Source: CAD feature listing. Evaluate the final solid. Frame: model axes, mm. Face numbers are marked on the shaded views. Give positions to 0.01 mm unless a question says otherwise; leave off trailing zeros. Order: outer loops, then holes, each group sorted by start corner. A loop starts at its lowest first (then second) coordinate and runs counter-clockwise, first axis right, second up. Notation, with made-up numbers: (-30.75, 55.5) - (-3.75, 55.5) arc R23 ccw to (-3.75, 79.5) - close; hole circle Ø6 at (-27.75, 15). An arc over 180 degrees is marked (long way). Write each question's results on one line, items separated by ' | '. Start each with the question number.
Item 1: Mould query, pull axis X, two halves, no side actions, for the marked faces 1, 2 and 3. Classes: released by +X, released by -X, zero draft, split by the parting line, or undercut.
Item 2: Contact query for a flat-ended pin moving along its axis: pin 1 Ø5 at (x, z) = (-0.5, 1.5) entering from -Y. Output: stop coordinate, or through.
Item 3: Section A-A on z = 0. Output: boundary loops of the cut face in (x, y), and give its area (3 significant figures).
Item 4: Section B-B on y = 1.7. Output: boundary loops of the cut face in (x, z), and give its area (3 significant figures).
Item 5: Line query: line 1 along X through (y, z) = (3.45, 0); line 2 along Z through (x, y) = (-1, 2.85); line 3 along Z through (x, y) = (0.5, 1.2). Output: solid intervals per line, ascending.
```python
from build123d import *

# Parameters (mm, degrees)
BODY_SKETCH_R   = 5
BODY_SKETCH_R_2 = 2.25
BODY_DEPTH      = 5
CHAMFERS_SIZE   = 0.4


with BuildPart() as part:
    # body_sketch → body (new body)
    with BuildSketch(Plane(origin=(0, 0, 0), x_dir=(1, 0, 0), z_dir=(0, 1, 0))):
        with Locations(Location((0, 0, 0), (0, 0, 270))):
            Circle(BODY_SKETCH_R)
        with Locations(Location((0, 0, 0), (0, 0, 270))):
            Circle(BODY_SKETCH_R_2, mode=Mode.SUBTRACT)
    extrude(amount=BODY_DEPTH)

    # chamfers
    chamfers_edges = [part.edges().sort_by_distance(p)[0] for p in [
        (0, 0, -5),
        (0, 5, -5),
        (0, 0, -2.25),
        (0, 5, -2.25),
    ]]
    chamfer(chamfers_edges, length=CHAMFERS_SIZE)


solid = part.part
```
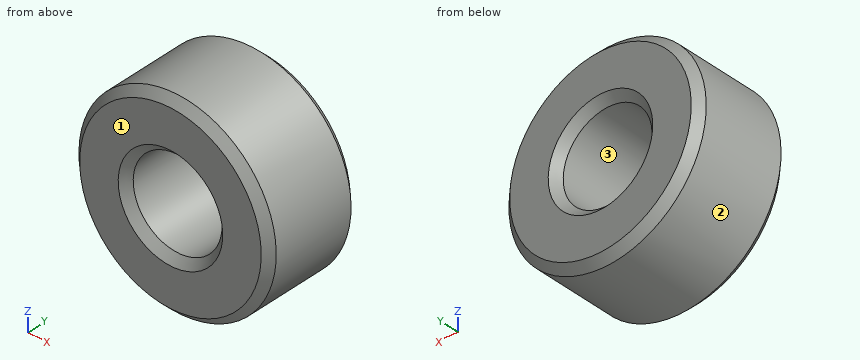
Evaluation:
1) face 1: zero draft | face 2: split by the parting line | face 3: undercut
2) pin 1: stops at y = 0
3) outline: (-5, 0.4) - (-4.6, 0) - (-2.65, 0) - (-2.25, 0.4) - (-2.25, 4.6) - (-2.65, 5) - (-4.6, 5) - (-5, 4.6) - close; (2.25, 0.4) - (2.65, 0) - (4.6, 0) - (5, 0.4) - (5, 4.6) - (4.6, 5) - (2.65, 5) - (2.25, 4.6) - close | area: 26.9 mm^2
4) outline: circle Ø10 at (0, 0); hole circle Ø4.5 at (0, 0) | area: 62.6 mm^2
5) line 1: x = -5 to -2.25, 2.25 to 5 | line 2: z = -4.9 to -2.02, 2.02 to 4.9 | line 3: z = -4.97 to -2.19, 2.19 to 4.97
